The listing builds one solid part. Answer for the finished solid, in the listing's coordinates (mm). A direction names the side the tool comes from. Give positions to 0.01 mm unless a question says otherwise; leave off trailing zeros. Order: outer loops, then holes, each group sorted by start corner. A loop starts at its lowest first (then second) coordinate and runs counter-clockwise, first axis right, second up. Notation, with made-up numbers: (3.5, 67.25) - (12.5, 67.25) arc R16 ccw to (12.5, 94.25) - close; hole circle Ø7 at (-32.75, -30). An arc over 180 degrees is marked (long way). Answer as a JSON object with one key per item and string values. Group by question number.
Q1. A cutting plane is placed at B-B, the plane z = 20. Give the vertices of the cut face in (x, y).
Q2. Consider line 1 (Z direction, x = 0, y = 0.85); line 2 (Z direction, x = 0, y = 4.1); line 3 (X direction, y = 11.5, z = 7.25). Determine where each line is inside the solid, lowest interval first.
Q3. The mould has two halves that part along Z. Classify faces 4 (the face through (-0.143, 4.276, 16.753)), 5 (the face through (4.51, 13.1, 14.35)), 6 (the face through (0, 9, 0)), 7 (the face through (0, 6, 14)): released by +Z, released by -Z, zero draft, split by the parting line, or undercut.
Q4. Given pin 1 (4 mm diameter, centred on x = 0, z = 20, fed in from +Y); pin 2 (1 mm diameter, centred on y = 11.5, z = 20.5, fed in from -X); pin 3 (5 mm diameter, centred on x = -3, y = 12.5, fed in from +Z); pin 4 (3.5 mm diameter, centred on x = -1, y = 13, fed in from +Z), each flat-ended and moving along its own axis, determine where each tip first touches the part or whether it passes through.
Q5. A cutting plane is placed at C-C, the plane y = 16. Give the vertices of the cut face in (x, z).
Q6. A cutting plane is placed at A-A, the plane x = 0. Give the vertices of the cut face in (y, z), and give its area (3 significant figures).
Q7. A cutting plane is placed at D-D, the plane x = -2.5. Give the vertices of the cut face in (y, z), and give its area (3 significant figures).
Q8. For faces 1 (the face through (1.4, 2.6, 21.4)), 2 (the face through (0, 13, 4)), 3 (the face through (1.03, 1.28, 6.65)), determine the directions among +Z, -Z, +X, -X, +Y, -Y from which every point of the face is accessible in a straight line to the end or side of a thin tool.
Autodesk Inventor part; units mm, degrees
ref_plane "YZ Plane" through (0, 0, 0) normal (1, 0, 0) x (0, 1, 0)
ref_plane "XZ Plane" through (0, 0, 0) normal (0, 1, 0) x (-1, 0, 0)
ref_plane "XY Plane" through (0, 0, 0) normal (0, 0, 1) x (1, 0, 0)
sketch "Skizze1" plane through (0, 0, 0) normal (1, 0, 0) x (0, 1, 0)
  line L0 (0, 30) -> (0, -5)
  line L1 (-4, 0) -> (24, 0)
  line L2 (0, 25) -> (0, 0)
  line L3 (0, 0) -> (20, 0)
  line L4 (20, 0) -> (20, 4)
  line L5 (20, 4) -> (6, 4)
  line L6 (6, 4) -> (6, 25)
  line L7 (6, 25) -> (0, 25)
  dimension "d0" = 20
  dimension "d1" = 25
  dimension "d2" = 4
  dimension "d3" = 6
extrude "Extrusion1" add sketch "Skizze1" along normal mid plane 11
sketch "Skizze2" plane through (-5.5, 6, 25) normal (0, 1, 0) x (1, 0, 0)
  line L0 (5.5, 30) -> (5.5, -5)
  line L1 (11, 0) -> (0, 0)
  point P0 (5.5, 25)
  point P1 (5.5, 5)
  point P2 (5.5, 17)
  dimension "d6" = 5
  dimension "d14" = 12
hole "Bohrung1" at (0, 6, 20) at (0, 6, 8) direction (0, -1, 0) diameter 3.4 end through all counterbore diameter 6.5 counterbore depth 3.4
sketch "Skizze3" plane through (0, 0, 0) normal (1, 0, 0) x (0, 1, 0)
  line L0 (20, 4) -> (6, 4)
  line L1 (6, 25) -> (0, 25)
  line L2 (20, 4) -> (6, 25)
  line L3 (6, 25) -> (6, 4)
  line L4 (6, 4) -> (20, 4)
  point P0 (0, 0)
  point P1 (6, 4)
extrude "Extrusion2" add sketch "Skizze3" against normal blind 2 from surface at 5.5
mirror "Spiegeln1" about plane through (0, 0, 0) normal (1, 0, 0) of "Extrusion2"
fillet "Rundung2" radius 2 3 edges at (0, 20, 0) (5.5, 3, 25) (-5.5, 3, 25)
properties part number "27_Switch_Holder_X" material "PET-Kunststoff"
Reply:
{
 "1": {"outline": "(-5.5, 0) - (-1.7, 0) - (-1.7, 2.6) - (-3.25, 2.6) - (-3.25, 6) - (-3.5, 6) - (-3.5, 9.33) - (-5.5, 9.33) - close; (1.7, 0) - (5.5, 0) - (5.5, 9.33) - (3.5, 9.33) - (3.5, 6) - (3.25, 6) - (3.25, 2.6) - (1.7, 2.6) - close"},
 "2": {"line 1": "z = 0 to 6.3, 9.7 to 18.3, 21.7 to 25", "line 2": "z = 0 to 4.75, 11.25 to 16.75, 23.25 to 25", "line 3": "x = -5.5 to -3.5, 3.5 to 5.5"},
 "3": {"face 4": "undercut", "face 5": "released by +Z", "face 6": "released by -Z", "face 7": "zero draft"},
 "4": {"pin 1": "stops at y = 2.6", "pin 2": "passes through", "pin 3": "stops at z = 18.92", "pin 4": "stops at z = 4"},
 "5": {"outline": "(-5.5, 0) - (5.5, 0) - (5.5, 10) - (3.5, 10) - (3.5, 4) - (-3.5, 4) - (-3.5, 10) - (-5.5, 10) - close"},
 "6": {"outline": "(0, 0) - (18, 0) arc R2 ccw to (20, 2) - (20, 4) - (6, 4) - (6, 4.75) - (2.6, 4.75) - (2.6, 6.3) - (0, 6.3) - close; (0, 9.7) - (2.6, 9.7) - (2.6, 11.25) - (6, 11.25) - (6, 16.75) - (2.6, 16.75) - (2.6, 18.3) - (0, 18.3) - close; (0, 21.7) - (2.6, 21.7) - (2.6, 23.25) - (6, 23.25) - (6, 25) - (0, 25) - close", "area": "143 mm^2"},
 "7": {"outline": "(0, 0) - (18, 0) arc R2 ccw to (20, 2) - (20, 4) - (6, 4) - (6, 5.92) - (2.6, 5.92) - (2.6, 10.08) - (6, 10.08) - (6, 17.92) - (2.6, 17.92) - (2.6, 22.08) - (6, 22.08) - (6, 25) - (0, 25) - close", "area": "177 mm^2"},
 "8": {"face 1": "+Y", "face 2": "+Z, +Y", "face 3": "+Y, -Y"}
}
